Verification items for the finished model (mm, model axes). Face numbers are marked on the shaded views. A direction names the side the tool comes from. Give positions to 0.01 mm unless a question says otherwise; leave off trailing zeros. Write each loop counter-clockwise with the first axis right and the second up, starting at its lowest first coordinate (ties: lowest second). Pieces come first, ordered by that corner, then holes. Notation, with made-up numbers: M -35.5,84 L -28.5,84 A21 cw -28.5,99 Z; hole C 21.5,-27 d9. An arc over 180 degrees is marked long. Write item = value, one per line.
from build123d import *
from build123d.topology import SkipClean

# Parameters (mm, degrees)
SKETCH1_W                                           = 80
SKETCH1_H                                           = 80
BOSS_EXTRUDE1_DEPTH                                 = 10
SKETCH2_W                                           = 10
SKETCH2_H                                           = 80
BOSS_EXTRUDE2_DEPTH                                 = 70
CSK_FOR_M3_COUNTERSUNK_FLAT_HEAD_SCREW1_D           = 3.2
CSK_FOR_M3_COUNTERSUNK_FLAT_HEAD_SCREW1_CSINK_D     = 6.3
CSK_FOR_M3_COUNTERSUNK_FLAT_HEAD_SCREW1_CSINK_ANGLE = 90
CUT_EXTRUDE2_DEPTH                                  = 91
SKETCH7_R                                           = 11.5
CUT_EXTRUDE1_DEPTH                                  = 121
FILLET2_R                                           = 40
SKETCH12_R                                          = 3.625
BOSS_EXTRUDE3_DEPTH                                 = 10
BOSS_EXTRUDE4_START                                 = -7
SKETCH14_R                                          = 11.5
SKETCH14_R_2                                        = 4.5
BOSS_EXTRUDE4_DEPTH                                 = 3
CUT_EXTRUDE4_DEPTH                                  = 98.979589711
BOSS_EXTRUDE5_START                                 = -10
SKETCH15_R                                          = 11.5
SKETCH15_R_2                                        = 4.5
BOSS_EXTRUDE5_DEPTH                                 = 3


with BuildPart() as part:
    # Sketch1 → Boss-Extrude1 (new body)
    with BuildSketch(Plane(origin=(0, 0, 0), x_dir=(1, 0, 0), z_dir=(0, 1, 0))):
        Rectangle(SKETCH1_W, SKETCH1_H)
    extrude(amount=BOSS_EXTRUDE1_DEPTH)

    # Sketch2 → Boss-Extrude2 (add)
    with BuildSketch(Plane(origin=(0, 10, 0), x_dir=(1, 0, 0), z_dir=(0, 1, 0))):
        with Locations((35, 0)):
            Rectangle(SKETCH2_W, SKETCH2_H)
    boss_extrude2 = extrude(amount=BOSS_EXTRUDE2_DEPTH)

    # CSK for M3 Countersunk Flat Head Screw1 (through all)
    with Locations(Plane.ZY.offset(-30)):
        with Locations((-15.5, 60.5), (15.5, 60.5), (15.5, 29.5), (-15.5, 29.5)):
            CounterSinkHole(CSK_FOR_M3_COUNTERSUNK_FLAT_HEAD_SCREW1_D / 2, CSK_FOR_M3_COUNTERSUNK_FLAT_HEAD_SCREW1_CSINK_D / 2, counter_sink_angle=CSK_FOR_M3_COUNTERSUNK_FLAT_HEAD_SCREW1_CSINK_ANGLE)

    # Mirror1: Boss-Extrude2 across plane
    add(boss_extrude2.mirror(Plane(origin=(0, 0, 0), x_dir=(0, 0, 1), z_dir=(1, 0, 0))))

    # Sketch11 → Cut-Extrude2 (cut, through all)
    with BuildSketch(Plane(origin=(0, 10, 0), x_dir=(1, 0, 0), z_dir=(0, 1, 0))):
        with BuildLine():
            Line((-2.281035949, -1.75), (2.281035949, -1.75))
            ThreePointArc((2.281035949, -1.75), (2.722462429, -0.924025608), (2.875, 0))
            ThreePointArc((2.875, 0), (-0.924025608, 2.722462429), (-2.281035949, -1.75))
        make_face()
    extrude(amount=-CUT_EXTRUDE2_DEPTH, mode=Mode.SUBTRACT)

    # Sketch7 → Cut-Extrude1 (cut, through all)
    with BuildSketch(Plane(origin=(40, 0, 0), x_dir=(0, 0, -1), z_dir=(1, 0, 0))):
        with Locations((0, 45)):
            Circle(SKETCH7_R)
    extrude(amount=-CUT_EXTRUDE1_DEPTH, mode=Mode.SUBTRACT)

    # Fillet2
    fillet2_edges = [part.edges().sort_by_distance(p)[0] for p in [
        (35, 80, -40),
        (35, 80, 40),
        (-35, 80, 40),
        (-35, 80, -40),
    ]]
    fillet(fillet2_edges, radius=FILLET2_R - 0.0001)  # a hair under: the kernel refuses the full size

    # Sketch12 → Boss-Extrude3 (add)
    with BuildSketch(Plane.XZ):
        with Locations(Location((0, 0, 0), (0, 0, 270))):
            Circle(SKETCH12_R)
        with BuildLine():
            Line((-2.281035949, 1.75), (2.281035949, 1.75))
            ThreePointArc((2.281035949, 1.75), (0, -2.875), (-2.281035949, 1.75))
        make_face(mode=Mode.SUBTRACT)
    extrude(amount=BOSS_EXTRUDE3_DEPTH)

    # Sketch14 → Boss-Extrude4 (add)
    with BuildSketch(Plane(origin=(-30, 0, 0), x_dir=(0, 0, -1), z_dir=(1, 0, 0)).offset(BOSS_EXTRUDE4_START)):
        with Locations((0, 45)):
            Circle(SKETCH14_R)
        with Locations((0, 45)):
            Circle(SKETCH14_R_2, mode=Mode.SUBTRACT)
    extrude(amount=-BOSS_EXTRUDE4_DEPTH)

    # Sketch13 → Cut-Extrude4 (cut, through all)
    with SkipClean():  # the faces are left unmerged after this step: merging them gives an invalid solid
        with BuildSketch(Plane(origin=(0, 0, 0), x_dir=(-1, 0, 0), z_dir=(0, -1, 0))):
            with BuildLine():
                Line((40, -40), (40, 0))
                ThreePointArc((40, 0), (28.284271346, -28.284271149), (2.79e-07, -40))
                Line((2.79e-07, -40), (40, -40))
            make_face()
            with BuildLine():
                Line((40, 0), (40, 40))
                Line((40, 40), (2.4e-08, 40))
                ThreePointArc((2.4e-08, 40), (28.284271256, 28.284271239), (40, 0))
            make_face()
        extrude(amount=-CUT_EXTRUDE4_DEPTH, mode=Mode.SUBTRACT)

    # Sketch15 → Boss-Extrude5 (add)
    with SkipClean():  # the faces are left unmerged after this step: merging them gives an invalid solid
        with BuildSketch(Plane.ZY.offset(-30).offset(BOSS_EXTRUDE5_START)):
            with Locations(Location((0, 45, 0), (0, 0, 180))):
                Circle(SKETCH15_R)
            with Locations(Location((0, 45, 0), (0, 0, 270))):
                Circle(SKETCH15_R_2, mode=Mode.SUBTRACT)
        extrude(amount=BOSS_EXTRUDE5_DEPTH)


solid = part.part
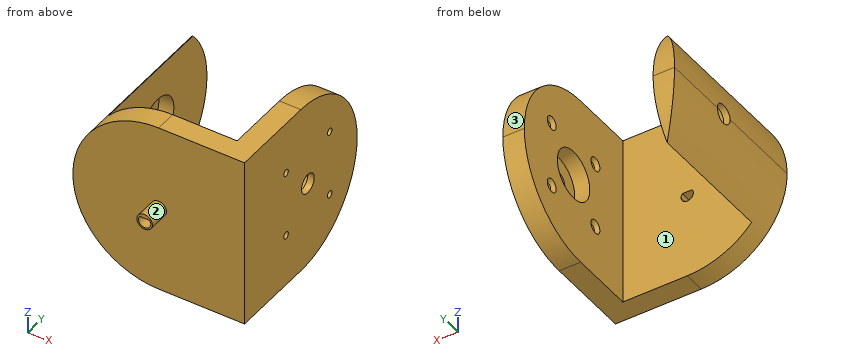
1) Cross-section at B-B on z = -15.5. Record the boundary of the cut face in (x, y).
From the geometry:
outline = M -36.87,0 L 40,0 L 40,27.9 L 31.55,27.9 L 30,26.35 L 30,10 L -30,10 L -30,76.87 L -36.87,76.87 Z; M 30,32.65 L 31.55,31.1 L 40,31.1 L 40,58.9 L 31.55,58.9 L 30,57.35 Z; M 30,63.65 L 31.55,62.1 L 40,62.1 L 40,76.87 L 30,76.87 Z
2) Depth check by flat-ended pin: P1, Ø6.5, axis at x = 0, z = 0, coming from the +Y side; P2, Ø3, axis at y = 60.5, z = 15.5, coming from the +X side; P3, Ø1.5, axis at x = 5.5, z = -30.5, coming from the -Y side. Enter the tip coordinate at first touch or a pass-through.
From the geometry:
P1 = 10
P2 = -30
P3 = 0
3) Cross-section at C-C on y = 74. Record the boundary of the cut face in (x, z), plus the area to 3 significant figures.
From the geometry:
outline = M -34,-21.07 L -30,-21.07 L -30,21.07 L -34,21.07 A40 ccw Z; M 30,-21.07 L 40,-21.07 L 40,21.07 L 30,21.07 Z
area = 761 mm^2
4) Cross-section at A-A on y = 29.5. Record the boundary of the cut face in (x, z), plus the area to 3 significant figures.
From the geometry:
outline = M -30,-26.46 L -30,26.46 A40 ccw Z; M 30,-40 L 40,-40 L 40,-17.1 L 31.55,-17.1 L 30,-18.65 Z; M 30,-12.35 L 31.55,-13.9 L 40,-13.9 L 40,13.9 L 31.55,13.9 L 30,12.35 Z; M 30,18.65 L 31.55,17.1 L 40,17.1 L 40,40 L 30,40 Z
area = 1,090 mm^2
5) Material ranges on probe 1 along Z at (x, y) = (35.25, 29.5); probe 2 along Y at (x, z) = (34.5, -15.5); probe 3 along Y at (x, z) = (-32, 0), recorded low to high. Write a range as from..to.
From the geometry:
probe_1 = -40..-17.1, -13.9..13.9, 17.1..40
probe_2 = 0..27.9, 31.1..58.9, 62.1..76.87
probe_3 = 0..33.5, 56.5..80
6) Tool access check on the marked faces 1, 2 and 3. Record the directions out of +Z, -Z, +X, -X, +Y, -Y that give a thin tool (end or side, any length) a straight path to the whole face; none if there is none.
From the geometry:
face_1 = +Z, -Z, +Y
face_2 = -Y
face_3 = +Z, +X, -X, +Y
7) Cross-section at D-D on x = 19.5. Record the boundary of the cut face in (y, z).
From the geometry:
outline = M 0,-40 L 10,-40 L 10,40 L 0,40 Z
